The model under review builds one solid part; all positions refer to its coordinate system, in mm. Face numbers are marked on the shaded views. A direction names the side the tool comes from. Give positions to 0.01 mm unless a question says otherwise; leave off trailing zeros. Order: outer loops, then holes, each group sorted by start corner. A loop starts at its lowest first (then second) coordinate and runs counter-clockwise, first axis right, second up. Notation, with made-up numbers: (56.5, -27) - (62.5, -27) arc R13 ccw to (62.5, -18) - close; hole circle Ø1 at (13, 20). An arc over 180 degrees is marked (long way). Use CSV: the item, a comma, the result in double quotes. Start each with the question number.
1. Take a section at B-B, the plane x = -5.75. State the section outline as (y, z) points.
2. Machinability: for the marked faces 1 and 2, which of the approach directions +Z, -Z, +X, -X, +Y, -Y give a long, thin tool a straight path to every point of the face, cutting with its end or side? Answer none if there is none.
3. Take a section at A-A, the plane z = 42.5. State the section outline as (x, y) points, then the cut area to 4 significant figures.
4. To check wall thickness, follow line 1 (Z direction, x = -0.9, y = 10.75); line 2 (Z direction, x = -1.25, y = 11.75); line 3 (Y direction, x = -0.8, z = -67.5). State the ranges of each line that lie inside material, in increasing order. Write a range as [from, to].
5. For pin 1 (2.5 mm diameter, centred on x = -5.75, z = 67.5, fed in from +Y); pin 2 (5.5 mm diameter, centred on y = 9, z = -7, fed in from -X); pin 3 (2.5 mm diameter, centred on x = -6, z = 22.5, fed in from +Y); pin 4 (0.8 mm diameter, centred on x = -1, z = -41.5, fed in from +Y), all flat-tipped, find the tip position at first contact; note any pin that passes through.
6. Take a section at C-C, the plane z = 22. State the section outline as (x, y) points.
Autodesk Inventor part; units mm, degrees
ref_plane "YZ Plane" through (0, 0, 0) normal (1, 0, 0) x (0, 1, 0)
ref_plane "XZ Plane" through (0, 0, 0) normal (0, 1, 0) x (-1, 0, 0)
ref_plane "XY Plane" through (0, 0, 0) normal (0, 0, 1) x (1, 0, 0)
sketch "Náčrt1" plane through (0, 0, 0) normal (0, 0, 1) x (1, 0, 0)
  line L0 (-10, 0) -> (0, 0)
  line L1 (0, 0) -> (0, 20)
  line L2 (0, 20) -> (-1.5, 20)
  line L3 (-1.5, 20) -> (-1.5, 1.5)
  line L4 (-1.5, 1.5) -> (-10, 1.5)
  line L5 (-10, 1.5) -> (-10, 0)
  line L6 (-12, 0) -> (2, 0)
  line L7 (0, 24) -> (0, -4)
  point P0 (0, 0)
  dimension "d0" = 20
  dimension "d1" = 10
  dimension "d2" = 1.5
  dimension "d3" = 1.5
extrude "Vysunutí1" add sketch "Náčrt1" along normal mid plane 145
sketch "Náčrt2" plane through (-10, 1.5, 72.5) normal (0, 1, 0) x (1, 0, 0)
  line L0 (0, 0) -> (0, 145)
  line L1 (8.5, 0) -> (0, 0)
  line L2 (8.5, 145) -> (8.5, 0)
  line L3 (0, 145) -> (8.5, 145)
  point P0 (10, 72.5)
  point P1 (4.25, 140)
  point P2 (4.25, 5)
  point P3 (4.25, 0)
  dimension "d6" = 4.25
  dimension "d7" = 4.25
  dimension "d57" = 5
  dimension "d78" = 5
hole "Díra1" at (-5.75, 1.5, -67.5) at (-5.75, 1.5, 67.5) direction (0, -1, 0) diameter 3.2 end through all
sketch "Náčrt9" plane through (-1.5, 1.5, 72.5) normal (-1, 0, 0) x (0, 0, 1)
  line L0 (-145, 18.5) -> (0, 18.5)
  line L1 (0, 18.5) -> (0, 0)
  point P0 (-72.5, -1.5)
  point P1 (-10, 9.25)
  point P2 (-30, 9.25)
  dimension "d79" = 9.25
  dimension "d80" = 9.25
  dimension "d81" = 10
  dimension "d82" = 30
hole "Díra7" at (-1.5, 10.75, 62.5) at (-1.5, 10.75, 42.5) direction (1, 0, 0) diameter 11 end through all
sketch "Náčrt10" plane through (0, 0, 72.5) normal (1, 0, 0) x (0, 0, -1)
  circle A0 centre (30, 10.75) radius 5.5
  circle A1 centre (10, 10.75) radius 5.5
  line L0 (145, 20) -> (0, 20)
  line L1 (0, 0) -> (0, 20)
  line L2 (145, 0) -> (0, 0)
  line L3 (145, 20) -> (145, 0)
  line L4 (60, 20) -> (136, 20)
  line L5 (136, 20) -> (136, 11)
  line L6 (136, 11) -> (60, 11)
  line L7 (60, 11) -> (60, 20)
  point P0 (72.5, 0)
  point P1 (60, 15.5)
  dimension "d90" = 76
  dimension "d91" = 9
  dimension "d92" = 60
extrude "Vysunutí3" cut sketch "Náčrt10" against normal through all contours L5 L6 L7 L0
sketch "Náčrt11" plane through (0, 0, 72.5) normal (1, 0, 0) x (0, 0, -1)
  line L0 (136, 20) -> (136, 11)
  line L1 (136, 11) -> (60, 11)
  line L2 (60, 11) -> (60, 20)
  line L3 (60, 20) -> (0, 20)
  line L4 (0, 0) -> (0, 20)
  line L5 (145, 0) -> (0, 0)
  line L6 (145, 20) -> (145, 0)
  line L7 (145, 20) -> (136, 20)
  circle A0 centre (10, 10.75) radius 5.5
  circle A1 centre (30, 10.75) radius 5.5
  point P0 (72.5, 0)
  point P1 (56, 15.5)
  point P2 (140, 15.5)
  point P3 (140.5, 20)
  point P4 (136, 15.5)
  dimension "d96" = 4.5
  dimension "d97" = 4
  dimension "d98" = 4.5
  dimension "d99" = 4
hole "Díra8" at (0, 15.5, 16.5) at (0, 15.5, -67.5) direction (-1, 0, 0) diameter 3.2 end through all
properties part number "panel" material "Hliník 6061"
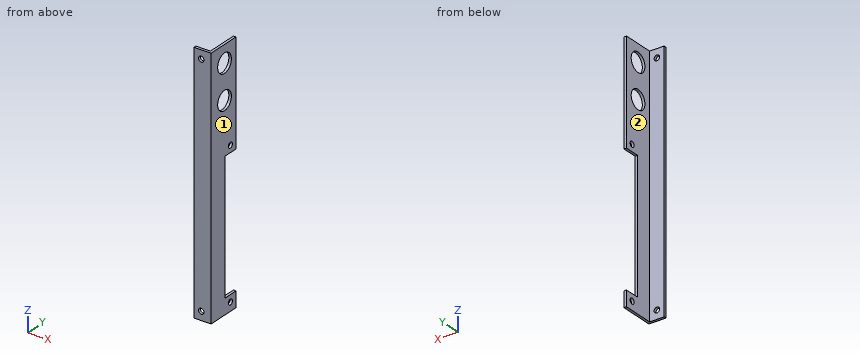
Determined:
1,outline,"(0, -72.5) - (1.5, -72.5) - (1.5, -69.1) - (0, -69.1) - close; (0, -65.9) - (1.5, -65.9) - (1.5, 65.9) - (0, 65.9) - close; (0, 69.1) - (1.5, 69.1) - (1.5, 72.5) - (0, 72.5) - close"
2,face 1,"+Z, -Z, +X, +Y, -Y"
2,face 2,"+Z, -Z, -X, +Y"
3,outline,"(-10, 0) - (0, 0) - (0, 5.25) - (-1.5, 5.25) - (-1.5, 1.5) - (-10, 1.5) - close; (-1.5, 16.25) - (0, 16.25) - (0, 20) - (-1.5, 20) - close"
3,area,"26.25 mm²"
4,line 1,"z = [-72.5, 37], [48, 57], [68, 72.5]"
4,line 2,"z = [-72.5, -63.5], [12.5, 37.09], [47.91, 57.09], [67.91, 72.5]"
4,line 3,"y = [0, 13.9], [17.1, 20]"
5,pin 1,"passes through"
5,pin 2,"stops at x = -1.5"
5,pin 3,"stops at y = 1.5"
5,pin 4,"stops at y = 11"
6,outline,"(-10, 0) - (0, 0) - (0, 20) - (-1.5, 20) - (-1.5, 1.5) - (-10, 1.5) - close"
